Here's how the part is built. I have some questions about the finished solid (model axes, mm). Face numbers are marked on the shaded views. A direction names the side the tool comes from. Give positions to 0.01 mm unless a question says otherwise; leave off trailing zeros. Loops run counter-clockwise (first coordinate to the right, second up) from the corner with the lowest first, then second, coordinate; pieces in that order, holes last.
Q1. I'm going to push flat-ended pins straight in: P1, Ø5, axis at x = -11, z = -20.5, coming from the +Y side; P2, Ø12, axis at x = 11, y = 19, coming from the +Z side; P3, Ø7.5, axis at y = 10, z = -10, coming from the +X side; P4, Ø16, axis at x = -10, z = -20, coming from the +Y side. Where does each tip first touch, or does it pass through?
Q2. Suppose I cut it at D-D (x = -14). List the corners of the cut face in (y, z) for me, and give its area (3 significant figures).
Q3. Suppose I cut it at B-B (x = 10). List the corners of the cut face in (y, z) for me, and give its area (3 significant figures).
Q4. For the marked faces 4 and 5, which set-ups out of +Z, -Z, +X, -X, +Y, -Y let a thin tool reach every point of the face, with its end or its side?
Q5. I need wall thicknesses on probe 1 along X at (y, z) = (28, -20); probe 2 along X at (y, z) = (13, -20); probe 3 along Z at (x, y) = (-7.5, 15). Which ranges of each line are inside material? Lowest first, please.
Q6. Suppose I cut it at A-A (y = 10). List the corners of the cut face in (x, z) for me.
Q7. Thinking about a two-plate mould opening in Z: for the marked faces 1, 2 and 3, which applies, pulls with the +Z half, pulls with the -Z half, needs draft (parallel to the pull), parting line crosses it, or undercut?
Q8. Suppose I cut it at C-C (z = -19). List the corners of the cut face in (x, y) for me.
Autodesk Inventor part; units mm, degrees
ref_plane "作業平面1" through (-18, 50, -30) normal (0, -1, 0) x (1, 0, 0)
ref_plane "YZ Plane" through (0, 0, 0) normal (1, 0, 0) x (0, 1, 0)
ref_plane "XZ Plane" through (0, 0, 0) normal (0, 1, 0) x (-1, 0, 0)
sketch "スケッチ1" plane through (0, 0, 0) normal (1, 0, 0) x (0, 1, 0)
  line L0 (0, 0) -> (15, 0)
  line L1 (15, 0) -> (36.0062, -30)
  line L2 (36.0062, -30) -> (0, -30)
  line L3 (0, -30) -> (0, 0)
  dimension "d0" = 35
  dimension "d1" = 15
  dimension "d2" = 30
extrude "押し出し1" add sketch "スケッチ1" along normal mid plane 36
ref_plane "作業平面1" through (-18, 50, -30) normal (0, -1, 0) x (1, 0, 0)
sketch "スケッチ3" plane through (-18, 50, -30) normal (0, -1, 0) x (1, 0, 0)
  line L0 (0, 0) -> (36, 0)
  line L1 (0, 30) -> (0, 0)
  line L2 (36, 0) -> (36, 30)
  point P0 (18, 30)
  point P1 (8, 10)
  point P2 (28, 10)
  dimension "d11" = 10
  dimension "d12" = 8
  dimension "d13" = 8
  dimension "d14" = 10
hole "穴1" at (-10, 50, -20) at (10, 50, -20) direction (0, -1, 0) diameter 5.5 end through all counterbore diameter 10 counterbore depth 30
sketch "スケッチ4" plane through (-18, 15, 0) normal (0, 0.8192, 0.5736) x (1, 0, 0)
  line L0 (18, 10) -> (18, 10)
  line L1 (18, 10) -> (18, 26.6232)
  line L2 (18, 26.6232) -> (18, 26.6232)
  line L3 (18, 26.6232) -> (18, 10)
  line L4 (0, 36.6232) -> (36, 36.6232)
  line L5 (0, 0) -> (36, 0)
  line L6 (0, 0) -> (0, 36.6232)
  line L7 (36, 36.6232) -> (36, 0)
  point P0 (18, -8.6036)
  dimension "d22" = 36.6232
  dimension "d24" = 10
  dimension "d36" = 10
  dimension "d46" = 18
  dimension "d47" = 18
  dimension "d51" = 36
hole "穴2" at (0, 30.2705, -21.8085) at (0, 20.7358, -8.1915) at (0, 30.2705, -21.8085) at (0, 20.7358, -8.1915) direction (0, -0.8192, -0.5736) diameter 5 depth 6 tip angle 118
sketch "スケッチ5" plane through (18, 0, 0) normal (1, 0, 0) x (0, 0, -1)
  circle A0 centre (10, 10) radius 6.05
  line L0 (0, 0) -> (30, 0)
  line L1 (0, 15) -> (0, 0)
  dimension "d40" = 10
  dimension "d41" = 10
  dimension "d42" = 12.1
extrude "押し出し3" cut sketch "スケッチ5" against normal through all
equation "\"d46\" = 0.5 * d51"
equation "\"d47\" = d46"
properties part number "s_base1"
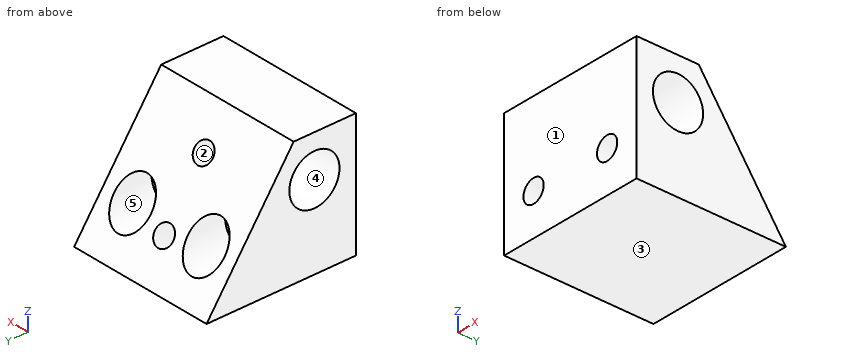
Solutions:
1. P1: stops at y = 20
1. P2: stops at z = 0
1. P3: passes through
1. P4: stops at y = 34.61
2. outline: (0, -30) - (36.01, -30) - (31.1, -23) - (20, -23) - (20, -17) - (26.9, -17) - (15, 0) - (0, 0) - close; hole circle Ø12.1 at (10, -10)
2. area: 596 mm2
3. outline: (0, -30) - (36.01, -30) - (32.51, -25) - (20, -25) - (20, -22.75) - (0, -22.75) - close; (0, -17.25) - (20, -17.25) - (20, -15) - (25.5, -15) - (15, 0) - (0, 0) - close; hole circle Ø12.1 at (10, -10)
3. area: 450 mm2
4. face 4: +X, -X
4. face 5: +Y
5. probe 1: x = -18 to -15, -5 to 5, 15 to 18
5. probe 2: x = -18 to -12.75, -7.25 to 7.25, 12.75 to 18
5. probe 3: z = -30 to -21.15, -18.85 to -13.41, -6.59 to 0
6. outline: (-18, -30) - (18, -30) - (18, -16.05) - (-18, -16.05) - close; (-18, -3.95) - (18, -3.95) - (18, 0) - (-18, 0) - close; hole circle Ø5.5 at (-10, -20); hole circle Ø5.5 at (10, -20)
7. face 1: needs draft
7. face 2: undercut
7. face 3: pulls with the -Z half
8. outline: (-18, 0) - (-12.56, 0) - (-12.56, 20) - (-14.9, 20) - (-14.9, 28.3) - (-18, 28.3) - close; (-7.44, 0) - (7.44, 0) - (7.44, 20) - (5.1, 20) - (5.1, 28.3) - (-5.1, 28.3) - (-5.1, 20) - (-7.44, 20) - close; (12.56, 0) - (18, 0) - (18, 28.3) - (14.9, 28.3) - (14.9, 20) - (12.56, 20) - close
